Autodesk Inventor part; units mm, degrees
ref_plane "YZ Plane" through (0, 0, 0) normal (1, 0, 0) x (0, 1, 0)
ref_plane "XZ Plane" through (0, 0, 0) normal (0, 1, 0) x (-1, 0, 0)
ref_plane "XY Plane" through (0, 0, 0) normal (0, 0, 1) x (1, 0, 0)
sketch "Sketch1" plane through (0, 0, 0) normal (0, 0, 1) x (1, 0, 0)
  line L0 (0, 0) -> (25, 0)
  line L1 (25, 0) -> (25, 40)
  line L2 (25, 40) -> (0, 40)
  line L3 (0, 40) -> (0, 0)
  dimension "d1" = 25
  dimension "d2" = 40
  dimension "d3" = 25
extrude "Extrusion1" add sketch "Sketch1" against normal blind 30
sketch "Sketch2" plane through (25, 0, 0) normal (1, 0, 0) x (0, 0, -1)
  line L0 (0, 0) -> (30, 0)
  circle A0 centre (15, 6.56) radius 2.46
extrude "Extrusion2" cut sketch "Sketch2" against normal blind 30
sketch "Sketch3" plane through (0, 0, 0) normal (-1, 0, 0) x (0, 0, 1)
  line L0 (0, 0) -> (-30, 0)
  line L1 (-25.05, 0) -> (-4.95, 0)
  line L2 (-4.95, 0) -> (-4.95, 33.12)
  line L3 (-4.95, 33.12) -> (-25.05, 33.12)
  line L4 (-25.05, 33.12) -> (-25.05, 0)
  dimension "d11" = 20.1
extrude "Extrusion3" cut sketch "Sketch3" against normal blind 20
sketch "Sketch4" plane through (0, 0, 0) normal (0, -1, 0) x (1, 0, 0)
  line L0 (20, -4.95) -> (20, -25.05)
  line L1 (20, -15) -> (25, -15)
  line L2 (25, 0) -> (25, -30)
  line L3 (20, -8.025) -> (25, -8.025)
  line L4 (25, -8.025) -> (25, -21.975)
  line L5 (25, -21.975) -> (20, -21.975)
  line L6 (20, -21.975) -> (20, -8.025)
  line L7 (20, -8.025) -> (25, -21.975) construction
  line L8 (25, -8.025) -> (20, -21.975) construction
  line L9 (25, -12.54) -> (25, -17.46)
  point P0 (0, 0)
  point P1 (22.5, -15)
  dimension "d14" = 13.95
extrude "Extrusion4" add sketch "Sketch4" along normal blind 15
sketch "Sketch5" plane through (20, 0, 0) normal (-1, 0, 0) x (0, 0, 1)
  circle A0 centre (-15, 6.56) radius 2.46
  circle A1 centre (-15, 6.56) radius 4.7025
  circle A2 centre (-15, 6.56) radius 2.46
  circle A3 centre (-15, 6.56) radius 2.46
  point P0 (0, 0)
  dimension "d17" = 9.405
extrude "Extrusion5" cut sketch "Sketch5" against normal blind 2.1
sketch "Sketch6" plane through (25, 0, 0) normal (1, 0, 0) x (0, 0, -1)
  circle A0 centre (15, 6.56) radius 4.7025
  line L0 (15, 6.56) -> (15, 23.56)
  circle A1 centre (15, 23.56) radius 2.46
  point P0 (0, 0)
  dimension "d20" = 17
  dimension "d21" = 4.92
extrude "Extrusion6" cut sketch "Sketch6" against normal blind 10 contours A1
sketch "Sketch7" plane through (20, 0, 0) normal (-1, 0, 0) x (0, 0, 1)
  circle A0 centre (-15, 23.56) radius 2.46
  circle A1 centre (-15, 23.56) radius 4.7025
  point P0 (0, 0)
  dimension "d24" = 9.405
extrude "Extrusion7" cut sketch "Sketch7" against normal blind 2.1
sketch "Sketch9" plane through (25, 0, 0) normal (1, 0, 0) x (0, 0, -1)
  circle A0 centre (15, 6.56) radius 2.46
  circle A1 centre (15, 6.56) radius 2.46
  circle A2 centre (15, 23.56) radius 2.46
  circle A3 centre (15, 23.56) radius 2.46
  line L0 (30, 40) -> (30, 0)
  line L1 (30, 0) -> (30, 40)
  line L2 (30, 40) -> (0, 40)
  line L3 (0, 40) -> (0, 0)
  line L4 (0, 0) -> (8.025, 0)
  line L5 (21.975, 0) -> (21.975, -15)
  line L6 (21.975, -15) -> (8.025, -15)
  line L7 (8.025, -15) -> (8.025, 0)
  line L8 (0, 0) -> (8.025, 0)
  line L9 (21.975, 0) -> (30, 0)
extrude "Extrusion8" add sketch "Sketch9" along normal blind 5
sketch "Sketch10" plane through (0, 40, 0) normal (0, 1, 0) x (1, 0, 0)
  line L0 (0, 30) -> (30, 30)
  line L1 (30, 0) -> (0, 0)
  line L2 (0, 30) -> (30, 30)
  line L3 (30, 30) -> (30, 0)
  line L4 (30, 0) -> (0, 0)
  line L5 (0, 0) -> (0, 30)
extrude "Extrusion9" add sketch "Sketch10" along normal blind 30
sketch "Sketch12" plane through (30, 0, 0) normal (1, 0, 0) x (0, 0, -1)
  circle A0 centre (15, 6.56) radius 2.46
  line L0 (15, 6.56) -> (15, 15.06)
  circle A1 centre (15, 15.06) radius 2.525
  point P0 (0, 0)
  dimension "d31" = 8.5
  dimension "d33" = 5.05
extrude "Extrusion10" cut sketch "Sketch12" against normal blind 30 contours A1
sketch "Sketch14" plane through (0, 0, 0) normal (0, 0, 1) x (1, 0, 0)
  line L0 (30, 70) -> (0, 70)
  line L1 (0, 70) -> (0, 85)
  line L2 (30, 0) -> (30, 70)
  line L3 (30, 100) -> (30, 70)
  line L4 (-12, 120) -> (15, 120)
  line L5 (-9.5, 118) -> (-7, 110)
  line L6 (-9.5, 118) -> (-12, 120)
  line L7 (-9.5, 102) -> (-7, 110)
  line L8 (-9.5, 102) -> (-12, 100)
  line L9 (30, 105) -> (15, 120)
  line L10 (30, 105) -> (30, 100)
  line L11 (0, 85) -> (0, 100)
  line L12 (0, 100) -> (-12, 100)
  point P0 (0, 0)
  dimension "d60" = 20
  dimension "d64" = 12
extrude "Extrusion12" add sketch "Sketch14" against normal blind 30
sketch "Sketch15" plane through (0, 0, -25.05) normal (-1, 0, 0) x (0, 0, 1)
  line L0 (0, 33.12) -> (20.1, 33.12)
  line L1 (20.1, 33.12) -> (20.1, 0)
  line L2 (0, 33.12) -> (20.1, 33.12)
  line L3 (20.1, 33.12) -> (20.1, 31.1)
  line L4 (20.1, 31.1) -> (0, 31.1)
  line L5 (0, 31.1) -> (0, 33.12)
  point P0 (25.05, 0)
  dimension "d57" = 2.02
extrude "Extrusion13" add sketch "Sketch15" against normal blind 20
properties part number "16mm_x_30mm"
Check sheet for the modelled part. Datum: model origin and axes. Units: mm. A direction names the side the tool comes from. Coordinates: 2 decimals unless noted, no trailing zeros. Loops run counter-clockwise (first coordinate to the right, second up) from the corner with the lowest first, then second, coordinate; pieces in that order, holes last. Notation, with made-up numbers: (23, 8.5) -> (45, 8.5) arc R13 cw to (45, 17.5) -> close; hole circle Ø3 at (29, 45.25). An arc over 180 degrees is marked (long way). Answer in a Markdown table with one row per item.
1. Material ranges on line 1 along Y through (x, z) = (22.5, -15) (3 decimals); line 2 along Y through (x, z) = (25.75, -15) (3 decimals); line 3 along Z through (x, y) = (28, 23.56), recorded low to high. Write a range as [from, to].
Check values:
| item | result |
|---|---|
| line 1 | y = [-15, 4.1], [9.02, 12.535], [17.585, 21.1], [26.02, 112.5] |
| line 2 | y = [-15, 4.1], [9.02, 12.535], [17.585, 21.1], [26.02, 109.25] |
| line 3 | z = [-30, -17.46], [-12.54, 0] |
2. Sectioned sample at B-B, the plane z = -15. Give the number of separate pieces and of enclosed holes in the cut face, then the cut area to 3 significant figures.
Check values:
| item | result |
|---|---|
| separate pieces | 4 |
| enclosed holes | 0 |
| area | 3,020 mm2 |
3. Go/stop test with flat-tipped pins: pin 1 (1 mm diameter, centred on x = 25, z = -6, fed in from +Y); pin 2 (4 mm diameter, centred on y = 48, z = -13.5, fed in from -X); pin 3 (3 mm diameter, centred on y = 8.5, z = -14, fed in from -X). Record where each tip stops, or that it passes through.
Check values:
| item | result |
|---|---|
| pin 1 | stops at y = 110.5 |
| pin 2 | stops at x = 0 |
| pin 3 | stops at x = 22.1 |
4. Release check for a two-part mould opening along Y. For faces 4 (the face through (10, 16, -25.05)), 5 (the face through (15, 0, -3)), 6 (the face through (25.995, 7.502, -17.272)) record: released by +Y, released by -Y, zero draft, split by the parting line, or undercut.
Check values:
| item | result |
|---|---|
| face 4 | zero draft |
| face 5 | released by -Y |
| face 6 | undercut |
5. Sectioned sample at A-A, the plane y = 23.56. Record the boundary of the cut face in (x, z).
Check values:
| item | result |
|---|---|
| outline | (0, -30) -> (30, -30) -> (30, -17.46) -> (22.1, -17.46) -> (22.1, -19.7) -> (20, -19.7) -> (20, -25.05) -> (0, -25.05) -> close; (0, -4.95) -> (20, -4.95) -> (20, -10.3) -> (22.1, -10.3) -> (22.1, -12.54) -> (30, -12.54) -> (30, 0) -> (0, 0) -> close |
6. Access from +Z, -Z, +X, -X, +Y, -Y to the whole of each face (thin tool, end or side, straight path). Record for faces 1 (the face through (-6, 100, -15)), 2 (the face through (18, 0, -27)), 3 (the face through (-8.27, 114.06, -14.79)).
Check values:
| item | result |
|---|---|
| face 1 | +Z, -Z, -X, -Y |
| face 2 | -Z, +X, -X, -Y |
| face 3 | +Z, -Z, -X |
7. Sectioned sample at D-D, the plane z = -2.5. Record the boundary of the cut face in (x, y).
Check values:
| item | result |
|---|---|
| outline | (-12, 100) -> (0, 100) -> (0, 0) -> (30, 0) -> (30, 105) -> (15, 120) -> (-12, 120) -> (-9.5, 118) -> (-7, 110) -> (-9.5, 102) -> close |
8. Sectioned sample at C-C, the plane x = 5. Record the boundary of the cut face in (y, z).
Check values:
| item | result |
|---|---|
| outline | (0, -30) -> (120, -30) -> (120, 0) -> (0, 0) -> (0, -4.95) -> (31.1, -4.95) -> (31.1, -25.05) -> (0, -25.05) -> close |
